```python
from build123d import *

# Parameters (mm, degrees)
BOSS_EXTRUDE1_DEPTH      = 1.5
BOSS_EXTRUDE1_DEPTH_BACK = 1.5
SKETCH1_R                = 12.5
SKETCH2_W                = 8
SKETCH2_H                = 2.6
CUT_EXTRUDE1_DEPTH       = 18.930421077
CUT_EXTRUDE2_DEPTH       = 18.693501632
CUT_EXTRUDE2_DEPTH_BACK  = 18.693501632


with BuildPart() as part:
    # Sketch1 → Boss-Extrude1 (new, two sides: drawn at the far end of the back side and taken through both)
    with BuildSketch(Plane(origin=(0, 0, 0), x_dir=(1, 0, 0), z_dir=(0, 1, 0)).offset(-BOSS_EXTRUDE1_DEPTH_BACK)):
        with Locations(Location((0, 0, 0), (0, 0, 270))):
            Circle(SKETCH1_R)
    extrude(amount=BOSS_EXTRUDE1_DEPTH + BOSS_EXTRUDE1_DEPTH_BACK)

    # Sketch2 → Cut-Extrude1 (cut, through all)
    with BuildSketch(Plane(origin=(0, 1.5, 0), x_dir=(1, 0, 0), z_dir=(0, 1, 0))):
        Polygon((9.375833025, 13.639419162), (5.375833025, 6.711215932), (3.124166975, 8.011215932), (7.124166975, 14.939419162), align=None)
        with Locations((12.5, 0)):
            Rectangle(SKETCH2_W, SKETCH2_H)
        Polygon((-7.124166975, 14.939419162), (-3.124166975, 8.011215932), (-5.375833025, 6.711215932), (-9.375833025, 13.639419162), align=None)
        with Locations((-12.5, 0)):
            Rectangle(SKETCH2_W, SKETCH2_H)
        Polygon((-9.375833025, -13.639419162), (-5.375833025, -6.711215932), (-3.124166975, -8.011215932), (-7.124166975, -14.939419162), align=None)
        Polygon((7.124166975, -14.939419162), (3.124166975, -8.011215932), (5.375833025, -6.711215932), (9.375833025, -13.639419162), align=None)
    extrude(amount=-CUT_EXTRUDE1_DEPTH, mode=Mode.SUBTRACT)

    # Sketch3 → Cut-Extrude2 (cut, two sides: drawn at the far end of the back side and taken through both)
    with BuildSketch(Plane(origin=(0, 0, 0), x_dir=(1, 0, 0), z_dir=(0, 1, 0)).offset(-CUT_EXTRUDE2_DEPTH_BACK)):
        with BuildLine():
            Line((-0.746821454, 1.5), (0.746821454, 1.5))
            ThreePointArc((0.746821454, 1.5), (2.246821454, 0), (0.746821454, -1.5))
            Line((0.746821454, -1.5), (-0.746821454, -1.5))
            ThreePointArc((-0.746821454, -1.5), (-2.246821454, 0), (-0.746821454, 1.5))
        make_face()
    extrude(amount=CUT_EXTRUDE2_DEPTH + CUT_EXTRUDE2_DEPTH_BACK, mode=Mode.SUBTRACT)


solid = part.part
```
Verification items for the finished model (mm, model axes). A direction names the side the tool comes from. Give positions to 0.01 mm unless a question says otherwise; leave off trailing zeros. Write each loop counter-clockwise with the first axis right and the second up, starting at its lowest first coordinate (ties: lowest second). Pieces come first, ordered by that corner, then holes. Notation, with made-up numbers: (-38.5, 1.25) - (-14.5, 1.25) arc R10 ccw to (-14.5, 19.25) - close; hole circle Ø8 at (38.5, 57). An arc over 180 degrees is marked (long way). Put each result on its own line as item: value.
Q1. Set-up check for faces 4 (the face through (-8.5, 0, 0)), 5 (the face through (6.345, 0.021, 8.39)), 6 (the face through (-6.345, 0.021, -8.39)), 7 (the face through (4.27, 0.02, -7.35)): record each of +Z, -Z, +X, -X, +Y, -Y from which the full face is reachable in a straight line by a thin tool's end or side.
Result:
face 4: -X, +Y, -Y
face 5: +Z, +Y, -Y
face 6: -Z, +Y, -Y
face 7: +Y, -Y
Q2. Scan lines: probe 1 along X at (y, z) = (0.4, 0); probe 2 along X at (y, z) = (0.85, 8.25); probe 3 along X at (y, z) = (-0.15, 8.5). Record each from-to range of solid material in increasing order. Write a range as from..to.
Result:
probe 1: -8.5..-2.25, 2.25..8.5
probe 2: -9.39..-6.26, -3.26..3.26, 6.26..9.39
probe 3: -9.17..-6.41, -3.41..3.41, 6.41..9.17
Q3. Mould release check, pull along Z, two halves, no side actions. Record for faces 1 (the face through (-3, 1.5, 0)), 2 (the face through (-4.234, 0.021, -7.37)), 3 (the face through (-10.86, -0.02, 6.19)): released by +Z, released by -Z, zero draft, split by the parting line, or undercut.
Result:
face 1: zero draft
face 2: undercut
face 3: released by +Z
Q4. Depth check by flat-ended pin: P1, Ø1.5, axis at x = -10, y = -0.5, coming from the +Z side; P2, Ø0.9, axis at x = -10, y = 0.5, coming from the -Z side; P3, Ø1.3, axis at y = 0.5, z = 0, coming from the +X side. Enter the tip coordinate at first touch or a pass-through.
Result:
P1: z = 8.41
P2: z = -8.07
P3: x = 8.5
Q5. Section check A-A on x = 10. Record the cut outline in (y, z), and give its area (3 significant figures).
Result:
outline: (-1.5, -7.5) - (1.5, -7.5) - (1.5, -1.3) - (-1.5, -1.3) - close; (-1.5, 1.3) - (1.5, 1.3) - (1.5, 7.5) - (-1.5, 7.5) - close
area: 37.2 mm2
Q6. Section check D-D on z = -9. Record the cut outline in (x, y), and give its area (3 significant figures).
Result:
outline: (-8.67, -1.5) - (-6.7, -1.5) - (-6.7, 1.5) - (-8.67, 1.5) - close; (-3.7, -1.5) - (3.7, -1.5) - (3.7, 1.5) - (-3.7, 1.5) - close; (6.7, -1.5) - (8.67, -1.5) - (8.67, 1.5) - (6.7, 1.5) - close
area: 34.0 mm2
Q7. Section check C-C on y = 0.9. Record the cut outline in (x, z).
Result:
outline: (-12.43, -1.3) arc R12.5 ccw to (-7.34, -10.12) - (-5.38, -6.71) - (-3.12, -8.01) - (-5.09, -11.42) arc R12.5 ccw to (5.09, -11.42) - (3.12, -8.01) - (5.38, -6.71) - (7.34, -10.12) arc R12.5 ccw to (12.43, -1.3) - (8.5, -1.3) - (8.5, 1.3) - (12.43, 1.3) arc R12.5 ccw to (7.34, 10.12) - (5.38, 6.71) - (3.12, 8.01) - (5.09, 11.42) arc R12.5 ccw to (-5.09, 11.42) - (-3.12, 8.01) - (-5.38, 6.71) - (-7.34, 10.12) arc R12.5 ccw to (-12.43, 1.3) - (-8.5, 1.3) - (-8.5, -1.3) - close; hole (-0.75, -1.5) - (0.75, -1.5) arc R1.5 ccw to (0.75, 1.5) - (-0.75, 1.5) arc R1.5 ccw to start
Q8. Section check B-B on z = 0. Record the cut outline in (x, y), and give its area (3 significant figures).
Result:
outline: (-8.5, -1.5) - (-2.25, -1.5) - (-2.25, 1.5) - (-8.5, 1.5) - close; (2.25, -1.5) - (8.5, -1.5) - (8.5, 1.5) - (2.25, 1.5) - close
area: 37.5 mm2
